Design review of the part built by this model. Coordinates are the model's own, in mm. Face numbers are marked on the shaded views. A direction names the side the tool comes from. Give positions to 0.01 mm unless a question says otherwise; leave off trailing zeros. Loops run counter-clockwise (first coordinate to the right, second up) from the corner with the lowest first, then second, coordinate; pieces in that order, holes last. Notation, with made-up numbers: (21, -23) -> (64, -23) arc R16 cw to (64, -6) -> close; hole circle Ø7 at (7.25, 7). An arc over 180 degrees is marked (long way). Use CSV: the item, a comma, the result in double quotes. Start each with the question number.
Item 1: We need section C-C (y = -11.75). State the section outline as (x, z) points, plus the area to 3 significant figures.
Item 2: Wall thickness on line 1 along X through (y, z) = (-6.5, 19.5); line 2 along Y through (x, z) = (13, 28.5); line 3 along Y through (x, z) = (13.5, 24.5): over which ranges is each line inside the solid? List them lowest first. Write a range as from..to.
Item 3: Clearance check with flat-ended pins moving along their axes: pin 1 (1.5 mm diameter, centred on y = -5.5, z = 20, fed in from -X); pin 2 (8 mm diameter, centred on x = 10.5, y = -9.5, fed in from +Z); pin 3 (8 mm diameter, centred on x = 20, z = 14, fed in from +Y). State where each tip first meets the part, or that it passes through.
Item 4: We need section B-B (z = 23). State the section outline as (x, y) points.
Item 5: We need section A-A (x = 15). State the section outline as (y, z) points.
Item 6: For the marked faces 1 and 2, list the 3-axis set-ups (+Z, -Z, +X, -X, +Y, -Y) from which the entire face can be reached by the end or side of a thin tool; tool diameter is ignored.
from build123d import *

# Parameters (mm, degrees)
F0_W     = 38.1
F0_H     = 31.75
F1_DEPTH = 25.4
F3_DEPTH = 25.4
F4_DEPTH = 0.0543467271


with BuildPart() as f1:
    # F0 (on Front) → F1 (new body)
    with BuildSketch(Plane.XZ):
        with Locations((19.05, 15.875)):
            Rectangle(F0_W, F0_H)
    extrude(amount=F1_DEPTH)

    # F2 (on Right) → F3 (cut)
    with BuildSketch(Plane.YZ):
        Polygon((0, 31.696639955), (-17.193024978, 32.0808403194), (0, 6.7235296592), align=None)
    extrude(amount=F3_DEPTH, mode=Mode.SUBTRACT)

    # F4 (cut, through all): a face of the model
    f4_faces = [f1.faces().sort_by_distance(p)[0] for p in [
        (12.7, -1.1939350803, 31.7233199775),
    ]]
    extrude(f4_faces, amount=-F4_DEPTH, mode=Mode.SUBTRACT)


solid = f1.part
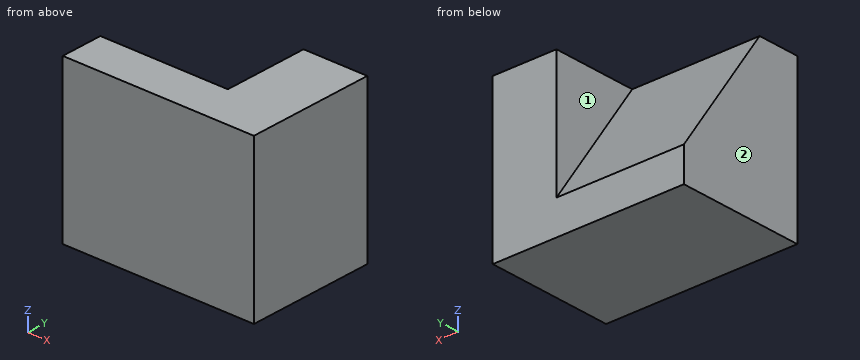
Results found:
1,outline,"(0, 0) -> (38.1, 0) -> (38.1, 31.75) -> (25.4, 31.75) -> (25.4, 24.05) -> (0, 24.05) -> close"
1,area,"1,010 mm²"
2,line 1,"25.4..38.1"
2,line 2,"-25.4..-14.77"
2,line 3,"-25.4..-12.05"
3,pin 1,"x = 25.4"
3,pin 2,"z = 26.63"
3,pin 3,"y = -2.22"
4,outline,"(0, -25.4) -> (38.1, -25.4) -> (38.1, 0) -> (25.4, 0) -> (25.4, -11.04) -> (0, -11.04) -> close"
5,outline,"(-25.4, 0) -> (0, 0) -> (0, 6.72) -> (-16.97, 31.75) -> (-25.4, 31.75) -> close"
6,face 1,"+Z, -X, +Y"
6,face 2,"+Z, -Z, -X, +Y, -Y"
